Input: part model. Units: mm. Frame: model coordinates. Coordinates: 2 decimals unless noted, no trailing zeros. Loops run counter-clockwise (first coordinate to the right, second up) from the corner with the lowest first, then second, coordinate; pieces in that order, holes last. Notation, with made-up numbers: (-4.5, 13) -> (7.5, 13) arc R12 cw to (7.5, 28) -> close; hole circle Ø5 at (67.5, -32). An arc over 180 degrees is marked (long way). Answer as a JSON object with one key per item and string values.
Autodesk Inventor part; units mm, degrees
ref_plane "YZ Plane" through (0, 0, 0) normal (1, 0, 0) x (0, 1, 0)
ref_plane "XZ Plane" through (0, 0, 0) normal (0, 1, 0) x (-1, 0, 0)
ref_plane "XY Plane" through (0, 0, 0) normal (0, 0, 1) x (1, 0, 0)
sketch "Sketch1" plane through (0, 0, 0) normal (1, 0, 0) x (0, 1, 0)
  line L0 (0, 0) -> (0, 15.24)
  line L1 (0, 0) -> (-101.6, 0) construction
  arc A0 (-101.6, 0) -> (0, 0) centre (-50.8, 607.4796) ccw
  line L2 (-50.8, -2.1204) -> (-50.8, 0) construction
  line L3 (0, 15.24) -> (101.6, 15.24) construction
  arc A1 (0, 15.24) -> (101.6, 15.24) centre (50.8, 622.7196) ccw construction
  line L4 (-101.6, 0) -> (-101.6, 15.24)
  line L5 (-101.6, 15.24) -> (0, 15.24)
  dimension "d0" = 15.24
  dimension "d1" = 101.6
  dimension "d3" = 50.8
  dimension "d4" = 2.1204
  dimension "d5" = 609.6
  dimension "d6" = 101.6
  dimension "d7" = 609.6
extrude "Extrusion1" add sketch "Sketch1" along normal mid plane 96.52
sketch "Sketch2" plane through (-48.26, -101.6, 15.24) normal (0, 0, 1) x (1, 0, 0)
  line L0 (48.26, 101.6) -> (48.26, 0) construction
  line L1 (0, 0) -> (96.52, 0) construction
  line L2 (0, 0) -> (0, 101.6) construction
  line L3 (0, 81.28) -> (96.52, 81.28) construction
  circle A0 centre (28.575, 81.28) radius 10.16
  circle A1 centre (67.945, 81.28) radius 7.62
  line L4 (0, 101.6) -> (96.52, 101.6)
  dimension "d11" = 20.32
  dimension "d12" = 15.24
  dimension "d13" = 57.15
  dimension "d14" = 19.685
  dimension "d20" = 20.32
extrude "Extrusion2" cut sketch "Sketch2" against normal through all
ref_plane "Work Plane1" through (-48.26, -20.32, 15.24) normal (0, 1, 0) x (1, 0, 0)
equation "\"d0\" = sidingDepth"
equation "\"d1\" = sidingHeight"
equation "\"d5\" = radiusOfCurvature"
equation "\"d6\" = sidingHeight"
equation "\"d7\" = radiusOfCurvature"
equation "\"d9\" = overallWidth"
equation "\"d11\" = leftPipeDiameter"
equation "\"d12\" = rightPipeDiameter"
equation "\"d13\" = outerDistanceBetweenPipep"
equation "\"d14\" = centerOfLeftPipe"
equation "\"d20\" = centerLineOfPipes"
equation "\"sidingHeight\" = 101.6"
equation "\"sidingDepth\" = 15.24"
equation "\"radiusOfCurvature\" = 609.6"
equation "\"centerLineOfPipes\" = 20.32"
equation "\"outerDistanceBetweenPipep\" = 57.15"
equation "\"leftPipeDiameter\" = 20.32"
equation "\"rightPipeDiameter\" = 15.24"
equation "\"overallWidth\" = 96.52"
equation "\"centerOfLeftPipe\" = 19.685"
equation "\"d21\" = -centerLineOfPipes"
properties part number "waterSoftenerDrainPipes"
1. Section query B-B (y = -20.32). Return loops of the section in (x, z) (3 decimals).
Reply:
{"outline": "(-48.26, -1.358) -> (-29.845, -1.358) -> (-29.845, 15.24) -> (-48.26, 15.24) -> close; (-9.525, -1.358) -> (12.065, -1.358) -> (12.065, 15.24) -> (-9.525, 15.24) -> close; (27.305, -1.358) -> (48.26, -1.358) -> (48.26, 15.24) -> (27.305, 15.24) -> close"}
2. Mould query, pull axis Y, two halves, no side actions, for faces 1 (the face through (48.26, -52, 7)), 2 (the face through (-0.68, -50.09, -2.12)), 3 (the face through (-9.994, -17.268, 6.848)). Classes: pulls with the +Y half, pulls with the -Y half, needs draft (parallel to the pull), parting line crosses it, or undercut.
Reply:
{"face 1": "needs draft", "face 2": "parting line crosses it", "face 3": "undercut"}
3. Line query: line 1 along X through (y, z) = (-20.32, 8.25) (3 decimals); line 2 along Y through (x, z) = (19.5, 14.5); line 3 along Y through (x, z) = (-17.5, 10). Output: solid intervals per line, ascending.
Reply:
{"line 1": "x = -48.26 to -29.845, -9.525 to 12.065, 27.305 to 48.26", "line 2": "y = -101.6 to -27.94, -12.7 to 0", "line 3": "y = -101.6 to -30.24, -10.4 to 0"}
4. Section query C-C (z = 4). Return loops of the section in (x, y) (3 decimals).
Reply:
{"outline": "(-48.26, -101.6) -> (48.26, -101.6) -> (48.26, 0) -> (-48.26, 0) -> close; hole circle Ø20.32 at (-19.685, -20.32); hole circle Ø15.24 at (19.685, -20.32)"}
5. Pin query (flat end, axial travel): P1, Ø13.5, axis at x = 19.685, y = -20.32, coming from the -Z side; P2, Ø10, axis at x = -37, z = 11.5, coming from the +Y side. Return the tip coordinate at first contact, or that it passes through.
Reply:
{"P1": "passes through", "P2": "stops at y = 0"}
6. Section query D-D (x = -14.5). Return loops of the section in (y, z).
Reply:
{"outline": "(-101.6, 0) arc R609.6 ccw to (-29.06, -1.73) -> (-29.06, 15.24) -> (-101.6, 15.24) -> close; (-11.58, -0.86) arc R609.6 ccw to (0, 0) -> (0, 15.24) -> (-11.58, 15.24) -> close"}
7. Section query A-A (x = -27). Return loops of the section in (y, z), plus the area to 3 significant figures.
Reply:
{"outline": "(-101.6, 0) arc R609.6 ccw to (-27.37, -1.67) -> (-27.37, 15.24) -> (-101.6, 15.24) -> close; (-13.27, -0.96) arc R609.6 ccw to (0, 0) -> (0, 15.24) -> (-13.27, 15.24) -> close", "area": "1,460 mm2"}
